Build history of the part. All positions in model axes, mm. A direction names the side the tool comes from. Give positions to 0.01 mm unless a question says otherwise; leave off trailing zeros. Write each loop counter-clockwise with the first axis right and the second up, starting at its lowest first coordinate (ties: lowest second). Pieces come first, ordered by that corner, then holes.
from build123d import *

# Parameters (mm, degrees)
SKETCH4_R           = 2.39
BOSS_EXTRUDE4_DEPTH = 3.18
BOSS_EXTRUDE5_DEPTH = 3.18


with BuildPart() as part:
    # Sketch4 → Boss-Extrude4 (new body)
    with BuildSketch(Plane.XY):
        with BuildLine():
            Line((-17.925296466, 35.419639483), (-17.925296466, 0.349476153))
            Line((-17.925296466, 0.349476153), (31.944623299, 0.349476153))
            Line((31.944623299, 0.349476153), (31.944623299, 34.287104082))
            ThreePointArc((31.944623299, 34.287104082), (29.279371809, 40.670159183), (22.886251145, 43.311175294))
            Line((22.886251145, 43.311175294), (-8.942333261, 43.311175294))
            ThreePointArc((-8.942333261, 43.311175294), (-14.920835694, 41.058088475), (-17.925296466, 35.419639483))
        make_face()
        with Locations((6.958119852, 31.252737949)):
            Circle(SKETCH4_R, mode=Mode.SUBTRACT)
        with Locations((6.958119852, 16.252738122)):
            Circle(SKETCH4_R, mode=Mode.SUBTRACT)
    extrude(amount=BOSS_EXTRUDE4_DEPTH)

    # Sketch2 → Boss-Extrude5 (add)
    with BuildSketch(Plane(origin=(0, 0, 0), x_dir=(1, 0, 0), z_dir=(0, 1, 0))):
        with BuildLine():
            Line((41.133140879, -45.477323382), (47.074703534, -45.477323382))
            ThreePointArc((47.074703534, -45.477323382), (54.145771346, -48.40625557), (57.074703534, -55.477323382))
            Line((57.074703534, -55.477323382), (57.074703534, -80.006057453))
            ThreePointArc((57.074703534, -80.006057453), (54.145771346, -87.077125264), (47.074703534, -90.006057453))
            Line((47.074703534, -90.006057453), (-32.925296466, -90.006057453))
            ThreePointArc((-32.925296466, -90.006057453), (-39.996364277, -87.077125264), (-42.925296466, -80.006057453))
            Line((-42.925296466, -80.006057453), (-42.925296466, -55.006057453))
            ThreePointArc((-42.925296466, -55.006057453), (-39.996364277, -47.934989641), (-32.925296466, -45.006057453))
            Line((-32.925296466, -45.006057453), (-27.800216568, -45.006057453))
            ThreePointArc((-27.800216568, -45.006057453), (-20.729148756, -42.077125264), (-17.800216568, -35.006057453))
            Line((-17.800216568, -35.006057453), (-17.800216568, -0.006057453))
            Line((-17.800216568, -0.006057453), (32.074703534, -0.006057453))
            Line((32.074703534, -0.006057453), (32.074703534, -36.418886037))
            ThreePointArc((32.074703534, -36.418886037), (34.727858406, -42.824168511), (41.133140879, -45.477323382))
        make_face()
    extrude(amount=BOSS_EXTRUDE5_DEPTH)


solid = part.part
(1) 3-axis set-ups, long thin cutter, end or side, ignore diameter. For faces 5 (the face through (54.22, 1.57, 87)), 6 (the face through (31.945, 17, 2)), 7 (the face through (-30, 2, 45.006)): which of +Z, -Z, +X, -X, +Y, -Y reach the whole face in a straight line?
(2) Mould opens along Z. For faces 1 (the face through (7, 43.311, 2)), 2 (the face through (-17.8, 2, 18)), 3 (the face through (-39.92, 1.57, 87.15)), 4 (the face through (7, 22, 0)) say: +Z half, -Z half, draft (parallel to the pull), parting line (faces both ways), or undercut.
(3) Saw through at B-B, the plane y = 6.5. List the corners of the cut face in (x, z).
(4) Drop flat-ended pins along their axis: pin 1 (6 mm diameter, centred on y = 7.5, z = 42.5, fed in from -X); pin 2 (1 mm diameter, centred on y = 12, z = 2, fed in from -X); pin 3 (5 mm diameter, centred on x = 7, z = 64.5, fed in from +Y); pin 4 (5.5 mm diameter, centred on x = 6.96, y = 16.25, fed in from +Z). Give the stop position or say it passes through.
(5) Probe line 1 (Y direction, x = -1, z = 6); line 2 (X direction, y = 2.5, z = 34.5). List the from-to ranges inside material, lowest first.
(6) Saw through at C-C, the plane z = 68. List the corners of the cut face in (x, y).
Computed values:
1. face 5: +Z, +X, +Y, -Y
1. face 6: +Z, -Z, +X, +Y
1. face 7: -Z, -X, +Y, -Y
2. face 1: draft
2. face 2: undercut
2. face 3: +Z half
2. face 4: -Z half
3. outline: (-17.93, 0) - (31.94, 0) - (31.94, 3.18) - (-17.93, 3.18) - close
4. pin 1: passes through
4. pin 2: stops at x = -17.93
4. pin 3: stops at y = 3.18
4. pin 4: stops at z = 3.18
5. line 1: y = 0 to 3.18
5. line 2: x = -17.8 to 32.07
6. outline: (-42.93, 0) - (57.07, 0) - (57.07, 3.18) - (-42.93, 3.18) - close
